For this review, take the finished solid that the model builds, in its own axes (mm). A direction names the side the tool comes from. Round coordinates to 2 decimals unless told otherwise and drop trailing zeros. Write item = value, one per line. Start each with the question number.
```python
from build123d import *

# Parameters (mm, degrees)
F2_R     = 4.5
F3_DEPTH = 2
F5_DEPTH = 1
F6_R     = 0.75


with BuildPart() as f1:
    # F0 (on Front) → F1 (revolve)
    with BuildSketch(Plane.XZ):
        with BuildLine():
            Line((0, 29.8004541546), (0, 0))
            Line((0, 0), (11.4705134183, 0))
            add(Edge.make_bspline(
                [(11.4705134183, 0), (11.732875476, 0.8153426281), (12.3002087209, 2.5784339199), (7.7813398519, 2.5139627986), (10.3795413858, 5.785382592), (5.7516333208, 4.1896015586), (4.58393068, 26.1483576562), (7.9913187248, 25.2292024384), (7.0513523289, 28.0690694522), (6.4515948717, 29.8004541546)],
                knots=[0, 0, 0, 0, 0.1067103807, 0.2298458507, 0.3357124996, 0.4373357909, 0.7615161745, 0.8492516397, 1, 1, 1, 1], degree=3))
            Line((6.4515948717, 29.8004541546), (0, 29.8004541546))
        make_face()
    revolve(axis=Axis((0, 0, 14.9002270773), (0, 0, 1)))

    # F2 (on face) → F3 (cut)
    with BuildSketch(Plane.XY.offset(29.8004541546)):
        Circle(F2_R)
    extrude(amount=-F3_DEPTH, mode=Mode.SUBTRACT)

    # F4 (on face) → F5 (cut)
    with BuildSketch(Plane.XY.offset(29.8004541546)):
        Polygon((1, 7.5), (-1, 7.5), (-1, 2.4142135624), (0, 1.4142135624), (1, 2.4142135624), align=None)
        Polygon((0, 1.4142135624), (-1, 2.4142135624), (-1, 1), (-0.4142135624, 1), align=None)
        Polygon((-1, 1), (-1, 2.4142135624), (-4.5961940777, 6.0104076401), (-6.0104076401, 4.5961940777), (-2.4142135624, 1), align=None)
        Polygon((4.5961940777, 6.0104076401), (1, 2.4142135624), (1, 1), (2.4142135624, 1), (6.0104076401, 4.5961940777), align=None)
        Polygon((1, 1), (1, 2.4142135624), (0, 1.4142135624), (0.4142135624, 1), align=None)
        Polygon((-1, 0.4142135624), (-1, 1), (-2.4142135624, 1), (-1.4142135624, 0), align=None)
        Polygon((2.4142135624, 1), (1, 1), (1, 0.4142135624), (1.4142135624, 0), align=None)
        Polygon((-1.4142135624, 0), (-2.4142135624, 1), (-7.5, 1), (-7.5, -1), (-2.4142135624, -1), align=None)
        Polygon((7.5, 1), (2.4142135624, 1), (1.4142135624, 0), (2.4142135624, -1), (7.5, -1), align=None)
        Polygon((-1, -1), (-1, -0.4142135624), (-1.4142135624, 0), (-2.4142135624, -1), align=None)
        Polygon((1.4142135624, 0), (1, -0.4142135624), (1, -1), (2.4142135624, -1), align=None)
        Polygon((-0.4142135624, -1), (-1, -1), (-1, -2.4142135624), (0, -1.4142135624), align=None)
        Polygon((-1, -2.4142135624), (-1, -1), (-2.4142135624, -1), (-6.0104076401, -4.5961940777), (-4.5961940777, -6.0104076401), align=None)
        Polygon((2.4142135624, -1), (1, -1), (1, -2.4142135624), (4.5961940777, -6.0104076401), (6.0104076401, -4.5961940777), align=None)
        Polygon((1, -2.4142135624), (1, -1), (0.4142135624, -1), (0, -1.4142135624), align=None)
        Polygon((0, -1.4142135624), (-1, -2.4142135624), (-1, -7.5), (1, -7.5), (1, -2.4142135624), align=None)
    extrude(amount=-F5_DEPTH, mode=Mode.SUBTRACT)

    # F6
    f6_edges = [f1.edges().sort_by_distance(p)[0] for p in [
        (-4.5, 0, 27.800454),
    ]]
    fillet(f6_edges, radius=F6_R)


solid = f1.part
```
1. Wall thickness on L1, parallel to Z at x = 3.25, y = -3.5; L2, parallel to Z at x = 1.5, y = -2.25; L3, parallel to Y at x = 1.5, z = 26.5: over which ranges is each line inside the solid? List them lowest first. Write a range as from..to.
2. Clearance check with flat-ended pins moving along their axes: pin 1 Ø0.9 at (x, y) = (-3.5, -3) entering from +Z; pin 2 Ø1.1 at (y, z) = (-5.5, 29) entering from +X; pin 3 Ø6 at (y, z) = (2, 21.5) entering from +X. State where each tip first meets the part, or that it passes through.
3. Machinability: for faces 1 (the flat face through (-6, -1, 29)), 2 (the flat face through (0, 6, 28.8)), 3 (the flat face through (4, -4, 28.8)), which of the approach directions +Z, -Z, +X, -X, +Y, -Y give a long, thin tool a straight path to every point of the face, cutting with its end or side? Answer none if there is none.
4. Draft analysis for pull direction X (two halves, no side actions). For faces 4 (the flat face through (0, 0, 27.8)), 5 (the flat face through (6, 0, 28.8)), state which applies: +X half, -X half, draft (parallel to the pull), parting line (faces both ways), or undercut.
Outcome:
q1.L1 = 0..28.8
q1.L2 = 0..27.8
q1.L3 = -7.23..7.23
q2.pin_1 = 28.8
q2.pin_2 = 4.61
q2.pin_3 = 5.86
q3.face_1 = +Z, +X, -X
q3.face_2 = +Z, +Y, -Y
q3.face_3 = +Z
q4.face_4 = undercut
q4.face_5 = draft
